from build123d import *

# Parameters (mm, degrees)
SKETCH_2_R          = 6
EXTRUDE_1_DEPTH     = 5
FILLET_2_R          = 10
SKETCH_3_R          = 4
CUT_EXTRUDE_1_DEPTH = 18


with BuildPart() as part:
    # 草图1 → 旋转1 (revolve)
    with BuildSketch(Plane.XY, mode=Mode.PRIVATE) as revolve_1_sk:
        Polygon((0, 0), (-13, 0), (-13, 5), (-15, 5), (-15, 8), (0, 8), align=None)
    revolve(revolve_1_sk.sketch.rotate(Axis((0, -267.914485955, 0), (0, 1, 0)), 180), axis=Axis((0, -267.914485955, 0), (0, 1, 0)))

    # 草图2 → 凸台-拉伸1 (add)
    with BuildSketch(Plane(origin=(0, 8, 0), x_dir=(1, 0, 0), z_dir=(0, 1, 0))):
        with Locations(Location((0, 0, 0), (0, 0, 180))):
            Circle(SKETCH_2_R)
    extrude(amount=EXTRUDE_1_DEPTH)

    # 圆角2
    # the kernel refuses this fillet: 10 mm, written as the material it adds along each edge
    with BuildSketch(Plane(origin=(0, 8, 0), x_dir=(-1, 0, 0), z_dir=(0, 0, -1))) as fillet_2_piece_1:
        with BuildLine():
            CenterArc((14.660254038, 10), FILLET_2_R, 210, 60)
            Line((6, 5), (6, 0))
            Line((6, 0), (14.660254038, 0))
        make_face()
    revolve(axis=Axis((0, 8, 0), (0, 1, 0)))

    # 草图3 → 切除-拉伸1 (cut)
    with BuildSketch(Plane(origin=(0, 13, 0), x_dir=(1, 0, 0), z_dir=(0, 1, 0))):
        with Locations(Location((0, 0, 0), (0, 0, 180))):
            Circle(SKETCH_3_R)
    extrude(amount=-CUT_EXTRUDE_1_DEPTH, mode=Mode.SUBTRACT)


solid = part.part
Design review of the part built by this model. Coordinates are the model's own, in mm. A direction names the side the tool comes from. Coordinates: 2 decimals unless noted, no trailing zeros. Order: outer loops, then holes, each group sorted by start corner. A loop starts at its lowest first (then second) coordinate and runs counter-clockwise, first axis right, second up.
Item 1: The part is to be moulded in two halves that separate along Z. For faces 3 (the flat face through (0.1, 5, -13.4)), 4 (the cylindrical face through (0.867, 6.591, -3.905)), 5 (the cylindrical face through (-10.316, 2.535, 7.91)), say which applies: pulls with the +Z half, pulls with the -Z half, needs draft (parallel to the pull), parting line crosses it, or undercut.
Item 2: Take a section at B-B, the plane x = 0. Write out the cut boundary in (y, z), then the cut area to 3 significant figures.
Item 3: For line 1 (Z direction, x = 0, y = 5.5); line 2 (Z direction, x = 0, y = 4); line 3 (X direction, y = 5.5, z = -2.25), list the stretches that pass through material, from the lowest coordinate up.
Item 4: For faces 1 (the flat face through (-3, 0, -3)), 2 (the flat face through (6.6, 8, 13.3)), list the 3-axis set-ups (+Z, -Z, +X, -X, +Y, -Y) from which the entire face can be reached by the end or side of a thin tool; tool diameter is ignored.
Item 5: For pin 1 Ø2 at (y, z) = (11.5, 6) entering from -X; pin 2 Ø12 at (x, z) = (5.5, 11) entering from +Y; pin 3 Ø3 at (x, z) = (-10, -6.5) entering from +Y, all flat-tipped, find the tip position at first contact; note any pin that passes through.
Item 6: Take a section at D-D, the plane y = 6. Write out the cut boundary in (x, z).
Item 7: Take a section at A-A, the plane z = 0. Write out the cut boundary in (x, y), then the cut area to 3 significant figures.
Item 8: Take a section at C-C, the plane y = 1.5. Write out the cut boundary in (x, z), then the cut area to 3 significant figures.
The answers:
1. face 3: needs draft
1. face 4: undercut
1. face 5: parting line crosses it
2. outline: (0, -13) - (5, -13) - (5, -15) - (8, -15) - (8, -14.66) arc R10 cw to (13, -6) - (13, -4) - (0, -4) - close; (0, 4) - (13, 4) - (13, 6) arc R10 cw to (8, 14.66) - (8, 15) - (5, 15) - (5, 13) - (0, 13) - close
2. area: 201 mm2
3. line 1: z = -15 to -4, 4 to 15
3. line 2: z = -13 to -4, 4 to 13
3. line 3: x = -14.83 to -3.31, 3.31 to 14.83
4. face 1: +Z, -Z, +X, -X, -Y
4. face 2: +Y
5. pin 1: stops at x = -5.67
5. pin 2: stops at y = 12.52
5. pin 3: stops at y = 8.94
6. outline: circle Ø30 at (0, 0); hole circle Ø8 at (0, 0)
7. outline: (-15, 5) - (-13, 5) - (-13, 0) - (-4, 0) - (-4, 13) - (-6, 13) arc R10 cw to (-14.66, 8) - (-15, 8) - close; (4, 0) - (13, 0) - (13, 5) - (15, 5) - (15, 8) - (14.66, 8) arc R10 cw to (6, 13) - (4, 13) - close
7. area: 201 mm2
8. outline: circle Ø26 at (0, 0); hole circle Ø8 at (0, 0)
8. area: 481 mm2
